```python
from build123d import *

# Parameters (mm, degrees)
F1_DEPTH = 10
F2_DEPTH = 2.5
F3_DEPTH = 1.5


# Not quite as in the source:
# - a feature names something its author has since deleted; it is built from what else it names


with BuildPart() as f1:
    # F0 (on Top) → F1 (new body)
    with BuildSketch(Plane.XY):
        with BuildLine():
            Line((-2.4494897428, 0.5), (2.4494897428, 0.5))
            ThreePointArc((2.4494897428, 0.5), (0, 2.5), (-2.4494897428, 0.5))
        make_face()
        with BuildLine():
            ThreePointArc((2.5, 0), (2.4873403825, 0.251272405), (2.4494897428, 0.5))
            Line((2.4494897428, 0.5), (-2.4494897428, 0.5))
            ThreePointArc((-2.4494897428, 0.5), (-2.5, 0), (-2.4494897428, -0.5))
            Line((-2.4494897428, -0.5), (2.4494897428, -0.5))
            ThreePointArc((2.4494897428, -0.5), (2.4873403825, -0.251272405), (2.5, 0))
        make_face()
        with BuildLine():
            ThreePointArc((-2.4494897428, -0.5), (0, -2.5), (2.4494897428, -0.5))
            Line((2.4494897428, -0.5), (-2.4494897428, -0.5))
        make_face()
    extrude(amount=-F1_DEPTH)

    # F0 (on Top) → F2 (join)
    with BuildSketch(Plane.XY):
        with BuildLine():
            ThreePointArc((-4.220485754, -0.5), (0, -4.25), (4.220485754, -0.5))
            Line((4.220485754, -0.5), (2.4494897428, -0.5))
            ThreePointArc((2.4494897428, -0.5), (0, -2.5), (-2.4494897428, -0.5))
            Line((-2.4494897428, -0.5), (-4.220485754, -0.5))
        make_face()
        with BuildLine():
            Line((2.4494897428, 0.5), (4.220485754, 0.5))
            ThreePointArc((4.220485754, 0.5), (0, 4.25), (-4.220485754, 0.5))
            Line((-4.220485754, 0.5), (-2.4494897428, 0.5))
            ThreePointArc((-2.4494897428, 0.5), (0, 2.5), (2.4494897428, 0.5))
        make_face()
        with BuildLine():
            Line((-2.4494897428, 0.5), (2.4494897428, 0.5))
            ThreePointArc((2.4494897428, 0.5), (0, 2.5), (-2.4494897428, 0.5))
        make_face()
        with BuildLine():
            ThreePointArc((-2.4494897428, -0.5), (0, -2.5), (2.4494897428, -0.5))
            Line((2.4494897428, -0.5), (-2.4494897428, -0.5))
        make_face()
    extrude(amount=F2_DEPTH)

    # F0 (on Top) → F3 (join)
    with BuildSketch(Plane.XY):
        with BuildLine():
            Line((-2.4494897428, 0.5), (-4.220485754, 0.5))
            ThreePointArc((-4.220485754, 0.5), (-4.25, 0), (-4.220485754, -0.5))
            Line((-4.220485754, -0.5), (-2.4494897428, -0.5))
            ThreePointArc((-2.4494897428, -0.5), (-2.5, 0), (-2.4494897428, 0.5))
        make_face()
        with BuildLine():
            ThreePointArc((2.5, 0), (2.4873403825, 0.251272405), (2.4494897428, 0.5))
            Line((2.4494897428, 0.5), (-2.4494897428, 0.5))
            ThreePointArc((-2.4494897428, 0.5), (-2.5, 0), (-2.4494897428, -0.5))
            Line((-2.4494897428, -0.5), (2.4494897428, -0.5))
            ThreePointArc((2.4494897428, -0.5), (2.4873403825, -0.251272405), (2.5, 0))
        make_face()
        with BuildLine():
            ThreePointArc((4.220485754, -0.5), (4.2426150223, -0.2504351666), (4.25, 0))
            ThreePointArc((4.25, 0), (4.2426150223, 0.2504351666), (4.220485754, 0.5))
            Line((4.220485754, 0.5), (2.4494897428, 0.5))
            ThreePointArc((2.4494897428, 0.5), (2.4873403825, 0.251272405), (2.5, 0))
            ThreePointArc((2.5, 0), (2.4873403825, -0.251272405), (2.4494897428, -0.5))
            Line((2.4494897428, -0.5), (4.220485754, -0.5))
        make_face()
    extrude(amount=F3_DEPTH)


solid = f1.part
```
The listing builds one solid part. Answer for the finished solid, in the listing's coordinates (mm). A direction names the side the tool comes from. Coordinates: 2 decimals unless noted, no trailing zeros. Write each loop counter-clockwise with the first axis right and the second up, starting at its lowest first coordinate (ties: lowest second). Pieces come first, ordered by that corner, then holes. Notation, with made-up numbers: (3, -11.5) - (18, -11.5) arc R28 ccw to (18, 15.5) - close; hole circle Ø2 at (53, 76). An arc over 180 degrees is marked (long way). Return JSON: item names as keys, results as strings. Group by question number.
Q1. Which of the six approach directions +Z, -Z, +X, -X, +Y, -Y give full straight-line access (tool end or side, diameter ignored) to faces 1 (the flat face through (2, -2, 0)), 2 (the flat face through (0, 0, 1.5)), 3 (the flat face through (0, -2, 2.5))?
Q2. The part is cut by section C-C on y = 1. Write down the section's boundary in (x, z).
Q3. Find the intervals of material crossed by line 1 along Z through (x, y) = (0.25, 3.5); line 2 along Z through (x, y) = (1.75, 0); line 3 along X through (y, z) = (1.5, 1.25), in increasing order. Write a range as [from, to].
Q4. The part is cut by section D-D on z = -4.5. Write down the section's boundary in (x, y), and give its area (3 significant figures).
Q5. The part is cut by section A-A on z = 1.75. Write down the section's boundary in (x, y), and give its area (3 significant figures).
Q6. The part is cut by section B-B on x = 2. Write down the section's boundary in (y, z), and give its area (4 significant figures).
Q7. Flat-ended cylindrical pins translate along their axes: pin 1 Ø1.1 at (x, z) = (-1.5, 2) entering from -Y; pin 2 Ø0.8 at (x, y) = (0, 0) entering from +Z; pin 3 Ø2 at (x, z) = (2.5, -2) entering from -Y. Find the tip coordinate at first contact, or state that the pin passes through.
Evaluation:
{
 "1": {"face 1": "-Z", "face 2": "+Z, +X, -X", "face 3": "+Z, +X, -X, +Y, -Y"},
 "2": {"outline": "(-4.13, 0) - (-2.29, 0) - (-2.29, -10) - (2.29, -10) - (2.29, 0) - (4.13, 0) - (4.13, 2.5) - (-4.13, 2.5) - close"},
 "3": {"line 1": "z = [0, 2.5]", "line 2": "z = [-10, 1.5]", "line 3": "x = [-3.98, 3.98]"},
 "4": {"outline": "circle Ø5 at (0, 0)", "area": "19.6 mm2"},
 "5": {"outline": "(-4.22, -0.5) arc R4.25 ccw to (4.22, -0.5) - close; (-4.22, 0.5) - (4.22, 0.5) arc R4.25 ccw to start", "area": "48.3 mm2"},
 "6": {"outline": "(-3.75, 0) - (-1.5, 0) - (-1.5, -10) - (1.5, -10) - (1.5, 0) - (3.75, 0) - (3.75, 2.5) - (0.5, 2.5) - (0.5, 1.5) - (-0.5, 1.5) - (-0.5, 2.5) - (-3.75, 2.5) - close", "area": "47.75 mm2"},
 "7": {"pin 1": "stops at y = -4.14", "pin 2": "stops at z = 1.5", "pin 3": "stops at y = -2"}
}
